Input: part model. Units: mm. Frame: model coordinates. Face numbers are marked on the shaded views. A direction names the side the tool comes from. Coordinates: 2 decimals unless noted, no trailing zeros. Write each loop counter-clockwise with the first axis right and the second up, starting at its lowest first coordinate (ties: lowest second). Pieces come first, ordered by that corner, then holes. Notation, with made-up numbers: M 71,37.5 L 100,37.5 A7 cw 100,43.5 Z; hole C 37,-2 d11. An arc over 180 degrees is marked long. Write each question's results on one line, items separated by ' | '. Start each with the question number.
1. Section query C-C, the plane z = 7. Output: boundary loops of the cut face in (x, y), and give its area (3 significant figures).
2. Pull-direction query (Z, two-part tool) for the marked faces 3, 4 and 5; classes: +Z half, -Z half, draft (parallel to the pull), parting line (faces both ways), or undercut.
3. First-contact query: pin 1 (1.5 mm diameter, centred on x = -1, z = 7, fed in from +Y); pin 2 (4 mm diameter, centred on x = 1, z = 0, fed in from +Y); pin 3 (1 mm diameter, centred on x = 4.5, y = -31, fed in from +Z). Flat tips, straight axial feed; report the tip coordinate or a pass-through.
4. Set-up query: the marked faces 1 and 2. Return all of +Z, -Z, +X, -X, +Y, -Y with unobstructed straight access to the full face (end or side cutting, diameter ignored); none if empty.
5. Section query A-A, the plane x = 0. Output: boundary loops of the cut face in (y, z).
6. Section query B-B, the plane z = 0. Output: boundary loops of the cut face in (x, y), and give its area (3 significant figures).
7. Ray query, probe 1 along Z at (x, y) = (0, -16.75); probe 2 along Y at (x, z) = (-8.25, 3); probe 3 along Z at (x, y) = (0.25, -50.5) (3 decimals). Return the intervals inside material, ascending.
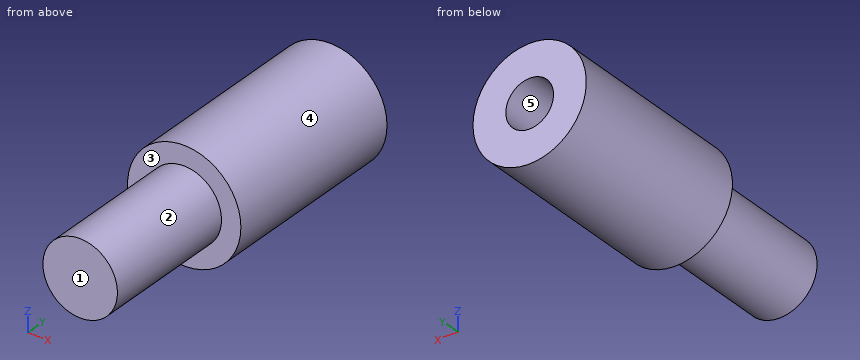
```python
from build123d import *

# Parameters (mm, degrees)
SKETCH_R     = 9.5
PAD_DEPTH    = 33
SKETCH001_R  = 4
POCKET_DEPTH = 30
SKETCH002_R  = 6.25
PAD001_DEPTH = 23.5


with BuildPart() as part:
    # Sketch → Pad (new body)
    with BuildSketch(Plane.XZ):
        Circle(SKETCH_R)
    extrude(amount=PAD_DEPTH)

    # Sketch001 (on Face2 of Pad) → Pocket (cut)
    with BuildSketch(Plane(origin=(0, 0, 0), x_dir=(1, 0, 0), z_dir=(0, 1, 0))):
        Circle(SKETCH001_R)
    extrude(amount=-POCKET_DEPTH, mode=Mode.SUBTRACT)

    # Sketch002 (on Face3 of Pocket) → Pad001 (join)
    with BuildSketch(Plane.XZ.offset(33)):
        Circle(SKETCH002_R)
    extrude(amount=PAD001_DEPTH)


solid = part.part
```
Answer:
1) outline: M -6.42,-33 L 6.42,-33 L 6.42,0 L -6.42,0 Z | area: 424 mm^2
2) face 3: draft | face 4: parting line | face 5: undercut
3) pin 1: y = 0 | pin 2: y = -30 | pin 3: z = 8.62
4) face 1: +Z, -Z, +X, -X, -Y | face 2: -Y
5) outline: M -56.5,-6.25 L -33,-6.25 L -33,-9.5 L 0,-9.5 L 0,-4 L -30,-4 L -30,4 L 0,4 L 0,9.5 L -33,9.5 L -33,6.25 L -56.5,6.25 Z
6) outline: M -9.5,-33 L -6.25,-33 L -6.25,-56.5 L 6.25,-56.5 L 6.25,-33 L 9.5,-33 L 9.5,0 L 4,0 L 4,-30 L -4,-30 L -4,0 L -9.5,0 Z | area: 681 mm^2
7) probe 1: -9.5 to -4, 4 to 9.5 | probe 2: -33 to 0 | probe 3: -6.245 to 6.245
